from build123d import *

# Parameters (mm, degrees)
SKETCH1_R                    = 2.600000007
BOSS_EXTRUDE1_DEPTH          = 6.35
BOSS_EXTRUDE2_DEPTH          = 12.446
SKETCH3_W                    = 74.675000002
SKETCH3_H                    = 34.925
BOSS_EXTRUDE4_DEPTH          = 12.446
SKETCH6_W                    = 12.446
SKETCH6_H                    = 57.212500002
BOSS_EXTRUDE5_DEPTH          = 9.525
SKETCH7_R                    = 1.650000002
CUT_EXTRUDE2_DEPTH           = 1
CUT_EXTRUDE2_DEPTH_BACK      = 45.196
SKETCH8_W                    = 9.525
SKETCH8_H                    = 6.35
BOSS_EXTRUDE6_DEPTH          = 12.446
SKETCH9_W                    = 1.524
SKETCH9_H                    = 9.525
CUT_EXTRUDE_THIN1_DEPTH      = 32.75
CUT_EXTRUDE_THIN1_DEPTH_BACK = 13.446
SKETCH10_R                   = 0.950000005
CUT_EXTRUDE3_DEPTH           = 12.262


with BuildPart() as part:
    # Sketch1 → Boss-Extrude1 (new body)
    with BuildSketch(Plane.XY):
        with BuildLine():
            Line((94.996, -31.75), (86.850341212, -31.75))
            ThreePointArc((86.850341212, -31.75), (78.719342976, -25.251372236), (70.104, -19.41004015))
            Line((70.104, -19.41004015), (70.104, -19.252396247))
            Line((70.104, -19.252396247), (70.104, 22.225))
            Line((70.104, 22.225), (70.104, 31.75))
            Line((70.104, 31.75), (101.6, 31.75))
            Line((101.6, 31.75), (101.6, 22.479))
            Line((101.6, 22.479), (94.996, 22.479))
            Line((94.996, 22.479), (94.996, -31.75))
        make_face()
        with Locations((88.9, -25.4)):
            Circle(SKETCH1_R, mode=Mode.SUBTRACT)
        with Locations((88.9, 25.4)):
            Circle(SKETCH1_R, mode=Mode.SUBTRACT)
    extrude(amount=BOSS_EXTRUDE1_DEPTH)

    # Sketch2 → Boss-Extrude2 (add)
    with BuildSketch(Plane.XY.offset(6.35)):
        Polygon((101.6, 22.479), (101.854, 22.479), (101.854, -31.75), (114.3, -31.75), (114.3, 31.75), (101.6, 31.75), align=None)
    extrude(amount=-BOSS_EXTRUDE2_DEPTH)

    # Sketch3 → Boss-Extrude4 (add)
    with BuildSketch(Plane(origin=(114.3, 0, 0), x_dir=(0, 0, -1), z_dir=(1, 0, 0))):
        Polygon((-6.35, -31.75), (-6.35, 22.225), (-87.375000002, 22.225), (-93.725000002, 22.225), (-93.725000002, -31.75), align=None)
        with Locations((-46.862500001, -4.7625)):
            Rectangle(SKETCH3_W, SKETCH3_H, mode=Mode.SUBTRACT)
    extrude(amount=-BOSS_EXTRUDE4_DEPTH)

    # Sketch6 → Boss-Extrude5 (add)
    with BuildSketch(Plane(origin=(0, 22.225, 0), x_dir=(1, 0, 0), z_dir=(0, 1, 0))):
        with Locations((108.077, -34.956250001)):
            Rectangle(SKETCH6_W, SKETCH6_H)
    extrude(amount=BOSS_EXTRUDE5_DEPTH)

    # Sketch7 → Cut-Extrude2 (cut, two sides)
    with BuildSketch(Plane(origin=(114.3, 0, 0), x_dir=(0, 0, -1), z_dir=(1, 0, 0))) as cut_extrude2_sk:
        with Locations((-88.962500002, -26.9875)):
            Circle(SKETCH7_R)
        with Locations((-46.862500001, -26.9875)):
            Circle(SKETCH7_R)
    extrude(amount=CUT_EXTRUDE2_DEPTH, mode=Mode.SUBTRACT)
    extrude(cut_extrude2_sk.sketch, amount=-CUT_EXTRUDE2_DEPTH_BACK, mode=Mode.SUBTRACT)

    # Sketch8 → Boss-Extrude6 (add)
    with BuildSketch(Plane(origin=(114.3, 0, 0), x_dir=(0, 0, -1), z_dir=(1, 0, 0))):
        with Locations((-79.437500002, 9.525)):
            Rectangle(SKETCH8_W, SKETCH8_H)
    extrude(amount=-BOSS_EXTRUDE6_DEPTH)

    # Sketch9 → Cut-Extrude-Thin1 (cut, two sides)
    with BuildSketch(Plane.ZY.offset(-101.854)) as cut_extrude_thin1_sk:
        with Locations((82.225000002, 17.4625)):
            Rectangle(SKETCH9_W, SKETCH9_H)
    extrude(amount=CUT_EXTRUDE_THIN1_DEPTH, mode=Mode.SUBTRACT)
    extrude(cut_extrude_thin1_sk.sketch, amount=-CUT_EXTRUDE_THIN1_DEPTH_BACK, mode=Mode.SUBTRACT)

    # Sketch10 → Cut-Extrude3 (cut)
    with BuildSketch(Plane.XY.offset(93.725000002)):
        with Locations((108.077, 14.700000064)):
            Circle(SKETCH10_R)
        with Locations((108.077, 18.224999872)):
            Circle(SKETCH10_R)
    extrude(amount=-CUT_EXTRUDE3_DEPTH, mode=Mode.SUBTRACT)


solid = part.part
Input: part model. Units: mm. Frame: model coordinates. A direction names the side the tool comes from. Coordinates: 2 decimals unless noted, no trailing zeros. Order: outer loops, then holes, each group sorted by start corner. A loop starts at its lowest first (then second) coordinate and runs counter-clockwise, first axis right, second up. Notation, with made-up numbers: M 10,46.25 L 54,46.25 A21 ccw 54,61.25 Z; hole C 24,4 d4. An arc over 180 degrees is marked long. Write item = value, one per line. Start each with the question number.
(1) Line query: line 1 along Z through (x, y) = (102, 0.5) (3 decimals); line 2 along Y through (x, z) = (88.9, 4); line 3 along X through (y, z) = (19.5, 66). Output: solid intervals per line, ascending. Write a range as [from, to].
(2) Section D-D on y = 25.4. Output: boundary loops of the cut face in (x, z), and give its area (3 significant figures).
(3) Section A-A on y = 8. Output: boundary loops of the cut face in (x, z) (3 decimals), and give its area (3 significant figures).
(4) Section B-B on z = 39.5. Output: boundary loops of the cut face in (x, y) (3 decimals), and give its area (3 significant figures).
(5) Reachability of faces 4 (the flat face through (101.6, 27, -3)), 5 (the flat face through (94.996, -4, 3)), 6 (the flat face through (108, 9, 74.675)), 7 (the flat face through (108, 17, 81.463)) from +Z, -Z, +X, -X, +Y, -Y: full face, straight path, thin tool, end or side. Return the list, or none.
(6) First-contact query: P1, Ø9.5, axis at x = 90, y = 0, coming from the +Z side; P2, Ø5, axis at y = 11, z = 83.5, coming from the -X side; P3, Ø0.8, axis at x = 105.5, z = 82, coming from the +Y side. Flat tips, straight axial feed; report the tip coordinate or a pass-through.
(7) Pull-direction query (Z, two-part tool) for faces 1 (the flat face through (108, 27, 63.563)), 2 (the flat face through (108, 6.35, 80)), 3 (the flat face through (108, 22.225, 88)); classes: released by +Z, released by -Z, zero draft, split by the parting line, or undercut.
(8) Section C-C on x = 88.9. Output: boundary loops of the cut face in (y, z), and give its area (3 significant figures).
Result set:
q1.line_1 = [-6.096, 9.525], [84.2, 93.725]
q1.line_2 = [-31.75, -28], [-22.8, 22.8], [28, 31.75]
q1.line_3 = [101.85, 114.3]
q2.outline = M 70.1,0 L 86.3,0 L 86.3,6.35 L 70.1,6.35 Z; M 91.5,0 L 101.6,0 L 101.6,-6.1 L 114.3,-6.1 L 114.3,63.56 L 101.85,63.56 L 101.85,6.35 L 91.5,6.35 Z
q2.area = 1,040 mm²
q3.outline = M 70.104,0 L 94.996,0 L 94.996,6.35 L 70.104,6.35 Z; M 101.854,-6.096 L 114.3,-6.096 L 114.3,9.525 L 101.854,9.525 Z; M 101.854,74.675 L 114.3,74.675 L 114.3,93.725 L 101.854,93.725 Z
q3.area = 590 mm²
q4.outline = M 101.854,-31.75 L 114.3,-31.75 L 114.3,-22.225 L 101.854,-22.225 Z; M 101.854,12.7 L 114.3,12.7 L 114.3,31.75 L 101.854,31.75 Z
q4.area = 356 mm²
q5.face_4 = -Z, -X, +Y, -Y
q5.face_5 = +Z, -Z, -Y
q5.face_6 = +X, -X
q5.face_7 = +X, -X, +Y
q6.P1 = 6.35
q6.P2 = 101.85
q6.P3 = 12.7
q7.face_1 = released by +Z
q7.face_2 = undercut
q7.face_3 = zero draft
q8.outline = M -31.75,0 L -28,0 L -28,6.35 L -31.75,6.35 Z; M -22.8,0 L 22.8,0 L 22.8,6.35 L -22.8,6.35 Z; M 28,0 L 31.75,0 L 31.75,6.35 L 28,6.35 Z
q8.area = 337 mm²
